The model under review builds one solid part; all positions refer to its coordinate system, in mm. A direction names the side the tool comes from. Coordinates: 2 decimals unless noted, no trailing zeros. Order: outer loops, then holes, each group sorted by start corner. A loop starts at its lowest first (then second) coordinate and runs counter-clockwise, first axis right, second up. Notation, with made-up numbers: M -8.5,54 L 15.5,54 A16 ccw 15.5,77 Z; hole C 76,-26.5 d8. An arc over 180 degrees is marked long. Write each question's results on one line, items separated by ' | '.
from build123d import *

# Parameters (mm, degrees)
SKETCH_R          = 7.18
PAD_DEPTH         = 24.325
SKETCH001_R       = 5.295
POCKET_DEPTH      = 0.15
SKETCH002_R       = 2.66
PAD001_DEPTH      = 1.37
PAD001_DEPTH_BACK = 1
SKETCH003_R       = 5.28
POCKET001_DEPTH   = 0.5
FILLET_R          = 1
FILLET001_R       = 0.3


with BuildPart() as part:
    # Sketch → Pad (new body, symmetric)
    with BuildSketch(Plane.XY):
        Circle(SKETCH_R)
    extrude(amount=PAD_DEPTH, both=True)

    # Sketch001 (on DatumPlane) → Pocket (cut)
    with BuildSketch(Plane.XY.offset(24.325)):
        Circle(SKETCH001_R)
    extrude(amount=-POCKET_DEPTH, mode=Mode.SUBTRACT)

    # Sketch002 (on DatumPlane) → Pad001 (join, two sides)
    with BuildSketch(Plane.XY.offset(24.325)) as pad001_sk:
        Circle(SKETCH002_R)
    extrude(amount=PAD001_DEPTH)
    extrude(pad001_sk.sketch, amount=-PAD001_DEPTH_BACK)

    # Sketch003 (on DatumPlane) → Pocket001 (cut)
    with BuildSketch(Plane.XY.offset(-24.325)):
        Circle(SKETCH003_R)
    extrude(amount=POCKET001_DEPTH, mode=Mode.SUBTRACT)

    # Fillet
    fillet_edges = [part.edges().sort_by_distance(p)[0] for p in [
        (-7.18, 0, 24.325),
        (-7.18, 0, -24.325),
    ]]
    fillet(fillet_edges, radius=FILLET_R)

    # Fillet001
    fillet001_edges = [part.edges().sort_by_distance(p)[0] for p in [
        (-2.66, 0, 25.695),
        (-2.66, 0, 24.175),
    ]]
    fillet(fillet001_edges, radius=FILLET001_R)


solid = part.part
1) To check wall thickness, follow line 1 along Z through (x, y) = (3, -0.5) (3 decimals); line 2 along X through (y, z) = (-0.25, 17); line 3 along Z through (x, y) = (5.5, 1.75) (3 decimals). State the ranges of each line that lie inside material, in increasing order.
Solutions:
line 1: -23.825 to 24.175 | line 2: -7.18 to 7.18 | line 3: -24.325 to 24.325
2) The part is to be moulded in two halves that separate along X. For faces 4 (the flat face through (5, 3, -24.325)), 5 (the flat face through (0, 0, -23.825)), 6 (the cylindrical face through (3.31, -6.37, 0.33)), say which applies: pulls with the +X half, pulls with the -X half, needs draft (parallel to the pull), parting line crosses it, or undercut.
Solutions:
face 4: needs draft | face 5: undercut | face 6: parting line crosses it
3) Take a section at C-C on z = 10.5. State the section outline as (x, y) points, plus the area to 3 significant figures.
Solutions:
outline: C 0,0 d14.36 | area: 162 mm2
4) For faces 1 (the cylindrical face through (-1.145, -5.154, -24.078)), 2 (the flat face through (0, 0, 25.695)), 3 (the flat face through (2.3, -2.3, 24.175)), list the 3-axis set-ups (+Z, -Z, +X, -X, +Y, -Y) from which the entire face can be reached by the end or side of a thin tool; tool diameter is ignored.
Solutions:
face 1: -Z | face 2: +Z, +X, -X, +Y, -Y | face 3: +Z
5) For pin 1 (3 mm diameter, centred on x = 3.5, z = -14.5, fed in from +Y); pin 2 (6 mm diameter, centred on y = -5.5, z = 13.5, fed in from +X); pin 3 (6.5 mm diameter, centred on x = 0, y = 0, fed in from -Z) (3 decimals), all flat-tipped, find the tip position at first contact; note any pin that passes through.
Solutions:
pin 1: y = 6.9 | pin 2: x = 6.73 | pin 3: z = -23.825
6) Take a section at A-A on y = 0. State the section outline as (x, z) points (3 decimals), plus the area to 3 significant figures.
Solutions:
outline: M -7.18,-23.325 A1 ccw -6.18,-24.325 L -5.28,-24.325 L -5.28,-23.825 L 5.28,-23.825 L 5.28,-24.325 L 6.18,-24.325 A1 ccw 7.18,-23.325 L 7.18,23.325 A1 ccw 6.18,24.325 L 5.295,24.325 L 5.295,24.175 L 2.96,24.175 A0.3 cw 2.66,24.475 L 2.66,25.395 A0.3 ccw 2.36,25.695 L -2.36,25.695 A0.3 ccw -2.66,25.395 L -2.66,24.475 A0.3 cw -2.96,24.175 L -5.295,24.175 L -5.295,24.325 L -6.18,24.325 A1 ccw -7.18,23.325 Z | area: 699 mm2
